Geometry check sheet. Reference: the model listing, model coordinates, mm. Coordinates: 2 decimals unless noted, no trailing zeros. Write each loop counter-clockwise with the first axis right and the second up, starting at its lowest first coordinate (ties: lowest second). Pieces come first, ordered by that corner, then holes. Notation, with made-up numbers: (46, 3.25) -> (77, 3.25) arc R19 ccw to (77, 14.25) -> close; hole circle Ø9 at (-7.5, 14.25). An arc over 180 degrees is marked (long way). Answer in a Markdown table with one row per item. Add a question column.
Q1. Section check B-B, the plane z = -145. Record the boundary of the cut face in (x, y), and give its area (3 significant figures).
Q2. Section check A-A, the plane z = -73. Record the boundary of the cut face in (x, y), and give its area (3 significant figures).
Q3. Section check C-C, the plane y = 1.95. Count the separate pieces of the cut face and the enclosed holes in it, and give its area (3 significant figures).
Q4. Thickness scan on line 1 (X direction, y = 1.2, z = -40); line 2 (X direction, y = 0.75, z = -32); line 3 (X direction, y = 1.4, z = -10.5). Record the ranges inside material, lowest first.
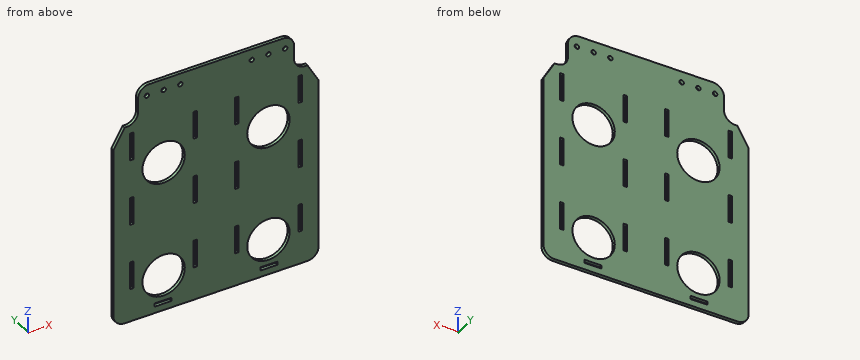
```python
from build123d import *

# Parameters (mm, degrees)
SKETCH_1_W          = 164
SKETCH_1_H          = 215
SKETCH_1_R          = 19
EXTRUDE_1_DEPTH     = 3
SKETCH_2_R          = 2
CUT_EXTRUDE_1_DEPTH = 3
SKETCH_3_W          = 3
SKETCH_3_H          = 25
CUT_EXTRUDE_2_DEPTH = 10
SKETCH_4_W          = 15
SKETCH_4_H          = 3
CUT_EXTRUDE_3_DEPTH = 10
SKETCH_6_W          = 10
SKETCH_6_H          = 190
EXTRUDE_2_DEPTH     = 3
CHAMFER_1_SIZE      = 25
CHAMFER_1_SIZE_2    = 14.43375673
FILLET_4_R          = 10
SKETCH_7_W          = 20
SKETCH_7_H          = 32.679491924
CUT_EXTRUDE_4_DEPTH = 10
FILLET_5_R          = 10
FILLET_6_R          = 10


with BuildPart() as part:
    # 草图1 → 凸台-拉伸1 (new body)
    with BuildSketch(Plane(origin=(0, 0, 0), x_dir=(1, 0, 0), z_dir=(0, 1, 0))):
        with Locations((47, 70)):
            Rectangle(SKETCH_1_W, SKETCH_1_H)
        with Locations(Location((94, 40, 0), (0, 0, 270))):
            Circle(SKETCH_1_R, mode=Mode.SUBTRACT)
        with Locations(Location((0, 40, 0), (0, 0, 270))):
            Circle(SKETCH_1_R, mode=Mode.SUBTRACT)
        with Locations(Location((0, 145, 0), (0, 0, 270))):
            Circle(SKETCH_1_R, mode=Mode.SUBTRACT)
        with Locations(Location((94, 145, 0), (0, 0, 270))):
            Circle(SKETCH_1_R, mode=Mode.SUBTRACT)
    extrude(amount=EXTRUDE_1_DEPTH)

    # 草图2 → 切除-拉伸1 (cut)
    with BuildSketch(Plane(origin=(0, 3, 0), x_dir=(1, 0, 0), z_dir=(0, 1, 0))):
        with Locations(Location((0, -27.5, 0), (0, 0, 270))):
            Circle(SKETCH_2_R)
        with Locations(Location((-15, -27.5, 0), (0, 0, 270))):
            Circle(SKETCH_2_R)
        with Locations(Location((15, -27.5, 0), (0, 0, 90))):
            Circle(SKETCH_2_R)
        with Locations(Location((79, -27.5, 0), (0, 0, 270))):
            Circle(SKETCH_2_R)
        with Locations(Location((109, -27.5, 0), (0, 0, 90))):
            Circle(SKETCH_2_R)
        with Locations(Location((94, -27.5, 0), (0, 0, 90))):
            Circle(SKETCH_2_R)
    extrude(amount=-CUT_EXTRUDE_1_DEPTH, mode=Mode.SUBTRACT)

    # 草图3 → 切除-拉伸2 (cut)
    with BuildSketch(Plane(origin=(0, 3, 0), x_dir=(1, 0, 0), z_dir=(0, 1, 0))):
        with Locations((28.5, 135)):
            Rectangle(SKETCH_3_W, SKETCH_3_H)
        with Locations((65.5, 135)):
            Rectangle(SKETCH_3_W, SKETCH_3_H)
        with Locations((28.5, 75)):
            Rectangle(SKETCH_3_W, SKETCH_3_H)
        with Locations((65.5, 75)):
            Rectangle(SKETCH_3_W, SKETCH_3_H)
        with Locations((28.5, 15)):
            Rectangle(SKETCH_3_W, SKETCH_3_H)
        with Locations((65.5, 15)):
            Rectangle(SKETCH_3_W, SKETCH_3_H)
        with Locations((-28.5, 15)):
            Rectangle(SKETCH_3_W, SKETCH_3_H)
        with Locations((-28.5, 75)):
            Rectangle(SKETCH_3_W, SKETCH_3_H)
        with Locations((-28.5, 135)):
            Rectangle(SKETCH_3_W, SKETCH_3_H)
        with Locations((122.5, 135)):
            Rectangle(SKETCH_3_W, SKETCH_3_H)
        with Locations((122.5, 75)):
            Rectangle(SKETCH_3_W, SKETCH_3_H)
        with Locations((122.5, 15)):
            Rectangle(SKETCH_3_W, SKETCH_3_H)
    extrude(amount=-CUT_EXTRUDE_2_DEPTH, mode=Mode.SUBTRACT)

    # 草图4 → 切除-拉伸3 (cut)
    with BuildSketch(Plane(origin=(0, 3, 0), x_dir=(1, 0, 0), z_dir=(0, 1, 0))):
        with Locations((-0.5, 170)):
            Rectangle(SKETCH_4_W, SKETCH_4_H)
        with Locations((94.5, 170)):
            Rectangle(SKETCH_4_W, SKETCH_4_H)
    extrude(amount=-CUT_EXTRUDE_3_DEPTH, mode=Mode.SUBTRACT)

    # 草图6 → 凸台-拉伸2 (add)
    with BuildSketch(Plane(origin=(0, 3, 0), x_dir=(1, 0, 0), z_dir=(0, 1, 0))):
        with Locations((-40, 82.5)):
            Rectangle(SKETCH_6_W, SKETCH_6_H)
        with Locations((134, 82.5)):
            Rectangle(SKETCH_6_W, SKETCH_6_H)
    extrude(amount=-EXTRUDE_2_DEPTH)

    # 倒角1
    # the kernel refuses this chamfer: 25, 14.43375673 mm, written as the material it takes off along each edge
    with BuildSketch(Plane(origin=(139, 67.677143866, 12.5), x_dir=(0.019326765612700705, 0, -0.9998132206222079), z_dir=(0, -1, 0))) as chamfer_1_piece_1_section:
        Polygon((CHAMFER_1_SIZE * 0.999813220622, -CHAMFER_1_SIZE * 0.0193267656127), (-CHAMFER_1_SIZE_2 * 0.0193267656124, -CHAMFER_1_SIZE_2 * 0.999813220604), (0, 0), align=None)
    chamfer_1_piece_1 = extrude(amount=132.354287732, mode=Mode.PRIVATE)
    chamfer_1_piece_1 = split(chamfer_1_piece_1, bisect_by=Plane(origin=(129, 1.5, 3.344472452), z_dir=(1, 0, 0)), keep=Keep.TOP, mode=Mode.PRIVATE)
    add(chamfer_1_piece_1, mode=Mode.SUBTRACT)
    with BuildSketch(Plane(origin=(-45, 67.677143866, 12.5), x_dir=(0.9983227437537926, 0, 0.057893862402670776), z_dir=(0, -1, 0))) as chamfer_1_piece_2_section:
        Polygon((CHAMFER_1_SIZE_2 * 0.998322743736, -CHAMFER_1_SIZE_2 * 0.0578938624016), (-CHAMFER_1_SIZE * 0.0578938624027, -CHAMFER_1_SIZE * 0.998322743754), (0, 0), align=None)
    chamfer_1_piece_2 = extrude(amount=132.354287732, mode=Mode.PRIVATE)
    chamfer_1_piece_2 = split(chamfer_1_piece_2, bisect_by=Plane(origin=(-35, 1.5, 3.344472452), z_dir=(-1, 0, 0)), keep=Keep.TOP, mode=Mode.PRIVATE)
    add(chamfer_1_piece_2, mode=Mode.SUBTRACT)

    # 圆角4
    fillet_4_edges = [part.edges().sort_by_distance(p)[0] for p in [
        (-35, 1.5, 37.5),
        (129, 1.5, 37.5),
        (-45, 1.5, -177.5),
        (139, 1.5, -177.5),
    ]]
    fillet(fillet_4_edges, radius=FILLET_4_R)

    # 草图7 → 切除-拉伸4 (cut)
    with BuildSketch(Plane(origin=(0, 3, 0), x_dir=(1, 0, 0), z_dir=(0, 1, 0))):
        with Locations((-33, -21.160254038)):
            Rectangle(SKETCH_7_W, SKETCH_7_H)
        with Locations((127, -21.160254038)):
            Rectangle(SKETCH_7_W, SKETCH_7_H)
    extrude(amount=-CUT_EXTRUDE_4_DEPTH, mode=Mode.SUBTRACT)

    # 圆角5
    fillet_5_edges = [part.edges().sort_by_distance(p)[0] for p in [
        (-23, 1.5, 37.5),
        (117, 1.5, 37.5),
    ]]
    fillet(fillet_5_edges, radius=FILLET_5_R)

    # 圆角6
    fillet_6_edges = [part.edges().sort_by_distance(p)[0] for p in [
        (-23, 1.5, 4.820508076),
        (117, 1.5, 4.820508076),
    ]]
    fillet(fillet_6_edges, radius=FILLET_6_R)


solid = part.part
```
Calculated:
| question | item | result |
|---|---|---|
| 1 | outline | (-45, 0) -> (-30, 0) -> (-30, 3) -> (-45, 3) -> close; (-27, 0) -> (-19, 0) -> (-19, 3) -> (-27, 3) -> close; (19, 0) -> (27, 0) -> (27, 3) -> (19, 3) -> close; (30, 0) -> (64, 0) -> (64, 3) -> (30, 3) -> close; (67, 0) -> (75, 0) -> (75, 3) -> (67, 3) -> close; (113, 0) -> (121, 0) -> (121, 3) -> (113, 3) -> close; (124, 0) -> (139, 0) -> (139, 3) -> (124, 3) -> close |
| 1 | area | 288 mm² |
| 2 | outline | (-45, 0) -> (-30, 0) -> (-30, 3) -> (-45, 3) -> close; (-27, 0) -> (27, 0) -> (27, 3) -> (-27, 3) -> close; (30, 0) -> (64, 0) -> (64, 3) -> (30, 3) -> close; (67, 0) -> (121, 0) -> (121, 3) -> (67, 3) -> close; (124, 0) -> (139, 0) -> (139, 3) -> (124, 3) -> close |
| 2 | area | 516 mm² |
| 3 | separate pieces | 1 |
| 3 | enclosed holes | 24 |
| 3 | area | 32,300 mm² |
| 4 | line 1 | x = -45 to -19, 19 to 75, 113 to 139 |
| 4 | line 2 | x = -45 to -17.23, 17.23 to 76.77, 111.23 to 139 |
| 4 | line 3 | x = -43.85 to -30, -27 to 27, 30 to 64, 67 to 121, 124 to 137.85 |
